from build123d import *

# Parameters (mm, degrees)
ESQUISSE1_R             = 10
ESQUISSE1_R_2           = 5
BOSS_EXTRU_1_DEPTH      = 5
ESQUISSE2_W             = 5
ESQUISSE2_H             = 7
BOSS_EXTRU_2_DEPTH      = 5
ESQUISSE3_R             = 1
ENL_V_MAT_EXTRU_1_DEPTH = 10


with BuildPart() as part:
    # Esquisse1 → Boss.-Extru.1 (new body)
    with BuildSketch(Plane.XY):
        Circle(ESQUISSE1_R)
        Circle(ESQUISSE1_R_2, mode=Mode.SUBTRACT)
    extrude(amount=BOSS_EXTRU_1_DEPTH)

    # Esquisse2 → Boss.-Extru.2 (add)
    with BuildSketch(Plane.XY.offset(5)):
        with Locations((0, 11.5)):
            Rectangle(ESQUISSE2_W, ESQUISSE2_H)
    boss_extru_2 = extrude(amount=-BOSS_EXTRU_2_DEPTH)

    # Esquisse3 → Enlèv. mat.-Extru.1 (cut)
    with BuildSketch(Plane(origin=(-2.5, 0, 0), x_dir=(0, -1, 0), z_dir=(-1, 0, 0))):
        with Locations((-12.345891544, 2.487364075)):
            Circle(ESQUISSE3_R)
    enl_v_mat_extru_1 = extrude(amount=-ENL_V_MAT_EXTRU_1_DEPTH, mode=Mode.SUBTRACT)

    # Symétrie1: Boss.-Extru.2, Enlèv. mat.-Extru.1 across plane
    add(boss_extru_2.mirror(Plane.ZX))
    add(enl_v_mat_extru_1.mirror(Plane.ZX), mode=Mode.SUBTRACT)


solid = part.part
The model under review builds one solid part; all positions refer to its coordinate system, in mm. A direction names the side the tool comes from. Give positions to 0.01 mm unless a question says otherwise; leave off trailing zeros. Write each loop counter-clockwise with the first axis right and the second up, starting at its lowest first coordinate (ties: lowest second). Pieces come first, ordered by that corner, then holes.
1. Add section A-A, the plane x = 0. Write out the cut boundary in (y, z), plus the area to 3 significant figures.
2. For P1, Ø1, axis at x = 8, y = 4.5, coming from the -Z side; P2, Ø1.5, axis at y = -12.5, z = 3, coming from the +X side; P3, Ø2, axis at y = -2.5, z = 2.5, coming from the -X side; P4, Ø2.5, axis at y = -12.35, z = 2.49, coming from the -X side, all flat-tipped, find the tip position at first contact; note any pin that passes through.
3. Add section B-B, the plane y = 0. Write out the cut boundary in (x, z), plus the area to 3 significant figures.
4. Wall thickness on L1, parallel to Y at x = 0, z = 3.65; L2, parallel to X at y = 0.25, z = 1.05; L3, parallel to Y at x = -0.5, z = 2.75: over which ranges is each line inside the solid? List them lowest first.
5. Add section D-D, the plane x = -3. Write out the cut boundary in (y, z).
6. Tool access review of faces 4 (the flat face through (2.5, 12, 4)), 5 (the flat face through (2.5, -12, 4)), 6 (the flat face through (-2.5, 12, 4)): name each direction out of +Z, -Z, +X, -X, +Y, -Y from which nothing blocks a thin tool from reaching the whole face with its end or side.
7. Add section C-C, the plane z = 3.1. Write out the cut boundary in (x, y), plus the area to 3 significant figures.
8. Draft analysis for pull direction Y (two halves, no side actions). For faces 1 (the flat face through (-2.5, -12, 4)), 2 (the cylindrical face through (-0.035, -11.392, 2.788)), 3 (the flat face through (0, 15, 3)), state which applies: +Y half, -Y half, draft (parallel to the pull), parting line (faces both ways), or undercut.
Worked answers:
1. outline: (-15, 0) - (-5, 0) - (-5, 5) - (-15, 5) - close; (5, 0) - (15, 0) - (15, 5) - (5, 5) - close; hole circle Ø2 at (-12.35, 2.49); hole circle Ø2 at (12.35, 2.49)
1. area: 93.7 mm2
2. P1: stops at z = 0
2. P2: stops at x = 2.5
2. P3: stops at x = -9.89
2. P4: stops at x = -2.5
3. outline: (-10, 0) - (-5, 0) - (-5, 5) - (-10, 5) - close; (5, 0) - (10, 0) - (10, 5) - (5, 5) - close
3. area: 50.0 mm2
4. L1: y = -15 to -5, 5 to 15
4. L2: x = -10 to -4.99, 4.99 to 10
4. L3: y = -15 to -13.31, -11.38 to -4.97, 4.97 to 11.38, 13.31 to 15
5. outline: (-9.54, 0) - (-4, 0) - (-4, 5) - (-9.54, 5) - close; (4, 0) - (9.54, 0) - (9.54, 5) - (4, 5) - close
6. face 4: +Z, -Z, +X, +Y
6. face 5: +Z, -Z, +X, -Y
6. face 6: +Z, -Z, -X, +Y
7. outline: (-2.5, -15) - (2.5, -15) - (2.5, -13.14) - (-2.5, -13.14) - close; (-2.5, -11.56) - (2.5, -11.56) - (2.5, -9.68) arc R10 ccw to (2.5, 9.68) - (2.5, 11.56) - (-2.5, 11.56) - (-2.5, 9.68) arc R10 ccw to (-2.5, -9.68) - close; (-2.5, 13.14) - (2.5, 13.14) - (2.5, 15) - (-2.5, 15) - close; hole circle Ø10 at (0, 0)
7. area: 271 mm2
8. face 1: draft
8. face 2: undercut
8. face 3: +Y half
